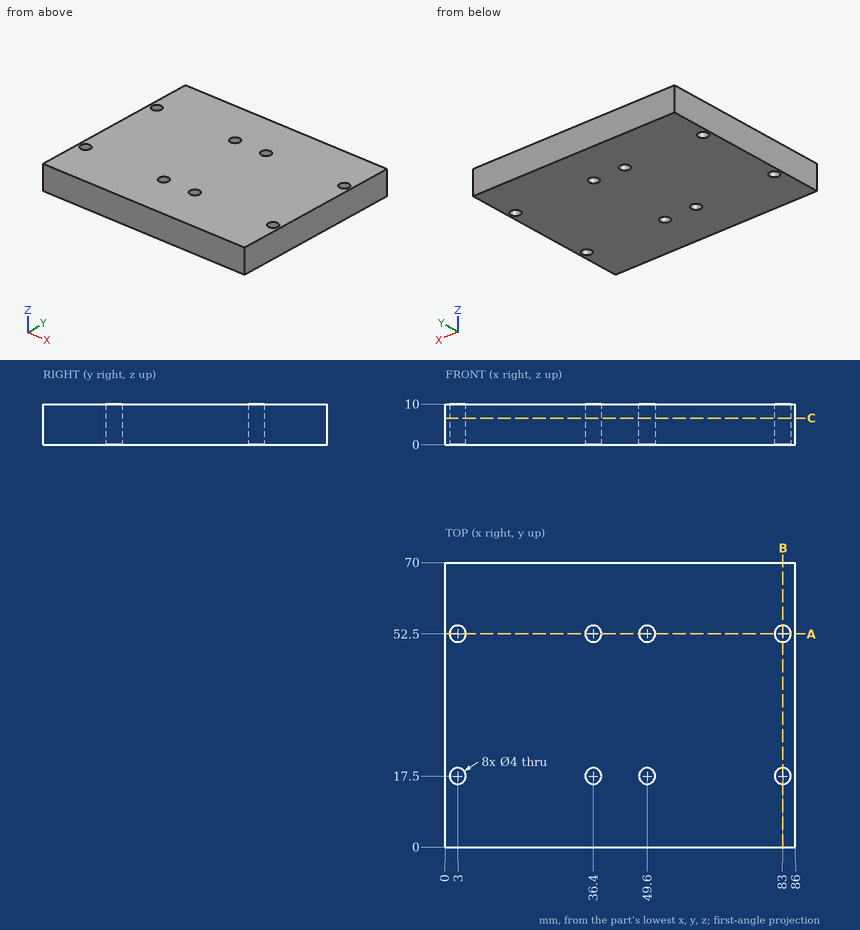
Geometry check sheet. Reference: drawing and pictorial views, mm from the part's lowest x, y, z. Give positions to 0.01 mm unless a question says otherwise; leave off trailing zeros. Order: outer loops, then holes, each group sorted by start corner. A loop starts at its lowest first (then second) coordinate and runs counter-clockwise, first axis right, second up. Notation, with made-up numbers: M 40.5,32 L 65.5,32 A27 cw 65.5,68 Z; hole C 55.25,61.5 d1. An arc over 180 degrees is marked long. Answer in a Markdown table with one row per item. Add a question column.
Item 1: Section check B-B, the plane x = 83. Enter the section's corners in (y, z).
Item 2: Section check C-C, the plane z = 6.5. State how many separate pieces and enclosed holes the cut face has, and give its area (3 significant figures).
Item 3: Scan lines: probe 1 along Y at (x, z) = (83, 3.5); probe 2 along X at (y, z) = (18.5, 2.25); probe 3 along Y at (x, z) = (4.5, 3). Record each from-to range of solid material in increasing order. Write a range as from..to.
Item 4: Section check A-A, the plane y = 52.5. Enter the section's corners in (x, z), and give its area (3 significant figures).
Filled sheet:
| question | item | result |
|---|---|---|
| 1 | outline | M 0,0 L 15.5,0 L 15.5,10 L 0,10 Z; M 19.5,0 L 50.5,0 L 50.5,10 L 19.5,10 Z; M 54.5,0 L 70,0 L 70,10 L 54.5,10 Z |
| 2 | separate pieces | 1 |
| 2 | enclosed holes | 8 |
| 2 | area | 5,920 mm^2 |
| 3 | probe 1 | y = 0..15.5, 19.5..50.5, 54.5..70 |
| 3 | probe 2 | x = 0..1.27, 4.73..34.67, 38.13..47.87, 51.33..81.27, 84.73..86 |
| 3 | probe 3 | y = 0..16.18, 18.82..51.18, 53.82..70 |
| 4 | outline | M 0,0 L 1,0 L 1,10 L 0,10 Z; M 5,0 L 34.4,0 L 34.4,10 L 5,10 Z; M 38.4,0 L 47.6,0 L 47.6,10 L 38.4,10 Z; M 51.6,0 L 81,0 L 81,10 L 51.6,10 Z; M 85,0 L 86,0 L 86,10 L 85,10 Z |
| 4 | area | 700 mm^2 |
